```python
from build123d import *

# Parameters (mm, degrees)
F1_DEPTH      = 101.6
F2_R          = 13.3499518003
F2_R_2        = 18.5793981889
F3_DEPTH      = 8.128
F3_DEPTH_BACK = 4.318
F5_START      = 94.742
F4_R          = 13.0989640124
F4_R_2        = 18.281744148
F5_DEPTH      = 13.97


with BuildPart() as f1:
    # F0 (on Right) → F1 (new body)
    with BuildSketch(Plane.YZ):
        Polygon((-21.862315014, 0), (-50.7084243, 0), (-110.2225035429, -28.0870012939), (166.6699335306, -28.0870012939), (150.910705328, 0), (102.6314273477, 0), align=None)
        Polygon((-10.5197704383, 29.3015744537), (-21.862315014, 0), (102.6314273477, 0), (91.0929739475, 29.3015744537), align=None)
    extrude(amount=F1_DEPTH)

    # F2 (on Right) → F3 (join, two sides)
    with BuildSketch(Plane.YZ) as f3_sk:
        with Locations((-54.4017069042, -28.1698741019)):
            Circle(F2_R)
        with Locations((102.5818586349, -28.1698741019)):
            Circle(F2_R_2)
    extrude(amount=-F3_DEPTH)
    extrude(f3_sk.sketch, amount=F3_DEPTH_BACK)

    # F4 (on Right) → F5 (join)
    with BuildSketch(Plane.YZ.offset(F5_START)):
        with Locations((-53.8203082979, -28.1698741019)):
            Circle(F4_R)
        with Locations((102.5559827685, -28.1698741019)):
            Circle(F4_R_2)
    extrude(amount=F5_DEPTH)


solid = f1.part
```
Work out the finished part from the listing and answer in its coordinate system (mm). A direction names the side the tool comes from. Give positions to 0.01 mm unless a question says otherwise; leave off trailing zeros. Order: outer loops, then holes, each group sorted by start corner. A loop starts at its lowest first (then second) coordinate and runs counter-clockwise, first axis right, second up.
1. For faces 4 (the flat face through (4.318, -55, -33)), 5 (the cylindrical face through (103.18, 110.99, -44.39)), 6 (the cylindrical face through (-3.38, 111.16, -44.65)), determine the directions among +Z, -Z, +X, -X, +Y, -Y from which every point of the face is accessible in a straight line to the end or side of a thin tool.
Result sheet:
face 4: -Z, +Y, -Y
face 5: +X
face 6: -X
2. Straight lines are drawn through the part: L1, parallel to X at y = 75, z = -22; L2, parallel to Z at x = 88.5, y = 52; L3, parallel to Z at x = 7, y = -49. For each, find the intervals that lie inside material, in ascending order.
Result sheet:
L1: x = 0 to 101.6
L2: z = -28.09 to 29.3
L3: z = -28.09 to 0
3. The mould has two halves that part along X. Classify faces 1 (the flat face through (0, 26, -5)), 2 (the flat face through (50, 26, -28.087)), 3 (the flat face through (50, -36, 0)): released by +X, released by -X, zero draft, split by the parting line, or undercut.
Result sheet:
face 1: released by -X
face 2: undercut
face 3: zero draft
4. Section C-C, the plane z = -22 is taken. Determine the outline of the cut face in (x, y), and give its area (3 significant figures).
Result sheet:
outline: (-8.13, -66.24) - (0, -66.24) - (0, -97.32) - (101.6, -97.32) - (101.6, -65.38) - (108.71, -65.38) - (108.71, -42.27) - (101.6, -42.27) - (101.6, 85.35) - (108.71, 85.35) - (108.71, 119.77) - (101.6, 119.77) - (101.6, 163.25) - (0, 163.25) - (0, 120.11) - (-8.13, 120.11) - (-8.13, 85.06) - (0, 85.06) - (0, -42.56) - (-8.13, -42.56) - close
area: 27,400 mm2
5. Section A-A, the plane z = -36 is taken. Determine the outline of the cut face in (x, y).
Result sheet:
outline: (-8.13, -65.21) - (4.32, -65.21) - (4.32, -43.59) - (-8.13, -43.59) - close; (-8.13, 85.73) - (4.32, 85.73) - (4.32, 119.43) - (-8.13, 119.43) - close; (94.74, -64.32) - (108.71, -64.32) - (108.71, -43.32) - (94.74, -43.32) - close; (94.74, 86.04) - (108.71, 86.04) - (108.71, 119.08) - (94.74, 119.08) - close
6. Each of these flat-tipped pins is pushed along its axis until it touches: P1, Ø2, axis at x = 61.5, y = -3, coming from the -Z side; P2, Ø4, axis at y = 82.5, z = 1, coming from the +X side; P3, Ø3, axis at x = 26, z = 8.5, coming from the +Y side. Where does it stop, or does it pass through?
Result sheet:
P1: stops at z = -28.09
P2: stops at x = 101.6
P3: stops at y = 99.87
7. Section D-D, the plane y = 19 is taken. Determine the outline of the cut face in (x, z).
Result sheet:
outline: (0, -28.09) - (101.6, -28.09) - (101.6, 29.3) - (0, 29.3) - close
8. Section B-B, the plane x = 47.5 is taken. Determine the outline of the cut face in (y, z).
Result sheet:
outline: (-110.22, -28.09) - (166.67, -28.09) - (150.91, 0) - (102.63, 0) - (91.09, 29.3) - (-10.52, 29.3) - (-21.86, 0) - (-50.71, 0) - close
